Here's the drawing with two shaded views (mm, measured from the low corner). I have some questions. A direction names the side the tool comes from. Coordinates: 2 decimals unless noted, no trailing zeros. Loops run counter-clockwise (first coordinate to the right, second up) from the corner with the lowest first, then second, coordinate; pieces in that order, holes last. Notation, with made-up numbers: (-12.75, 52) -> (-4.75, 52) arc R20 ccw to (-4.75, 90) -> close; hole circle Ø1 at (66.25, 73). An arc over 180 degrees is marked (long way). Answer as a JSON object with one key per item and string values. Group by question number.
Q1. I want a section at A-A on z = 17. Write out the boundary of the cut face in (x, y), then the cut area to 3 significant figures.
Q2. I want a section at C-C on z = 11. Write out the boundary of the cut face in (x, y), then the cut area to 3 significant figures.
Q3. I need wall thicknesses on line 1 (X direction, y = 31, z = 13.5); line 2 (Z direction, x = 5, y = 30); line 3 (Z direction, x = 11.5, y = 23). Which ranges of each line are inside material? Lowest first, please.
Q4. I want a section at D-D on y = 30. Write out the boundary of the cut face in (x, z).
Q5. I'm going to push flat-ended pins straight in: pin 1 (3 mm diameter, centred on x = 6, z = 10.5, fed in from -Y); pin 2 (1.5 mm diameter, centred on x = 15.5, y = 17, fed in from +Z); pin 3 (8 mm diameter, centred on x = 57.5, z = 24, fed in from +Y). Where does each tip first touch, or does it pass through?
Q6. Thinking about a two-plate mould opening in Y: for the marked faces 1, 2, 3 and 4, which applies, released by +Y, released by -Y, zero draft, split by the parting line, or undercut?
Q7. On a 3-axis mill with a long thin cutter (end or side, diameter ignored), from which of +Z, -Z, +X, -X, +Y, -Y can I reach the whole of each face in a straight line? I mean the marked faces 5, 6, 7, 8 and 9. Say none if no direction works.
Q8. I want a section at B-B on x = 30. Write out the boundary of the cut face in (y, z).
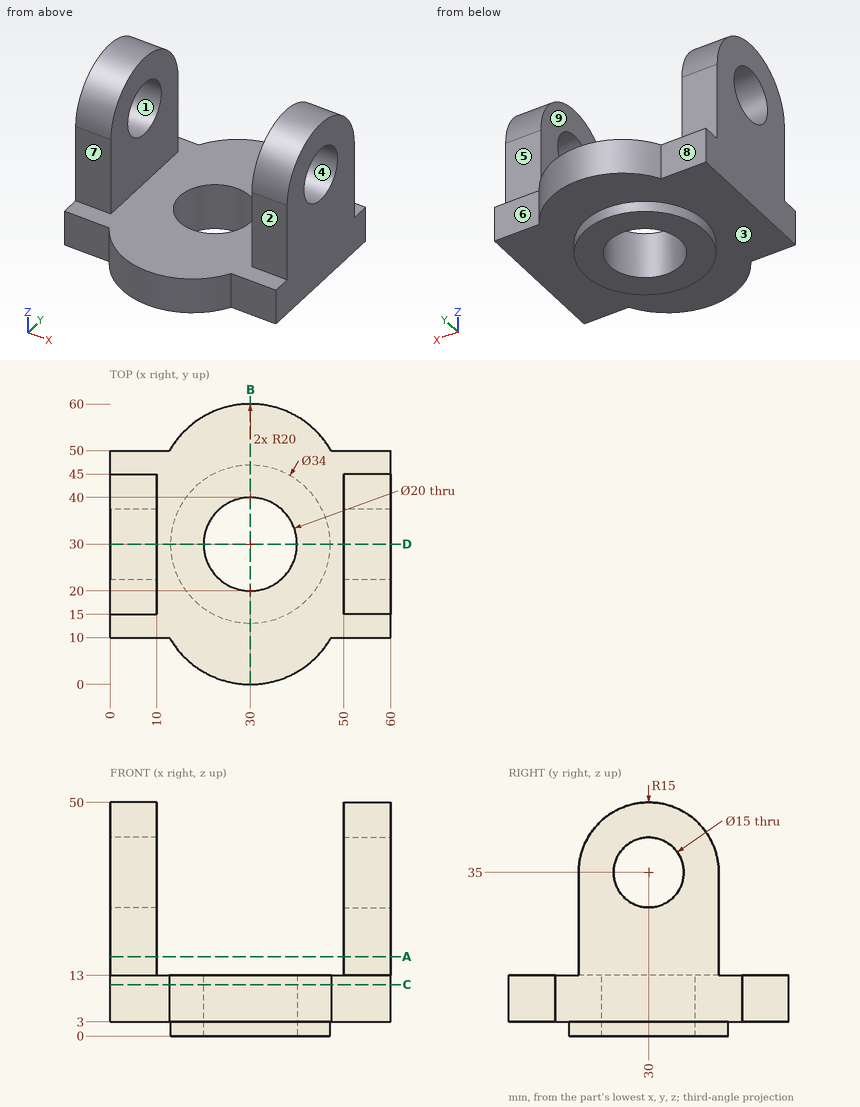
Result set:
{
 "1": {"outline": "(0, 15) -> (10, 15) -> (10, 45) -> (0, 45) -> close; (50, 15) -> (60, 15) -> (60, 45) -> (50, 45) -> close", "area": "600 mm²"},
 "2": {"outline": "(0, 10) -> (12.68, 10) arc R20 ccw to (47.32, 10) -> (60, 10) -> (60, 50) -> (47.32, 50) arc R20 ccw to (12.68, 50) -> (0, 50) -> close; hole circle Ø20 at (30, 30)", "area": "2,580 mm²"},
 "3": {"line 1": "x = 0 to 10, 50 to 60", "line 2": "z = 3 to 27.5, 42.5 to 50", "line 3": "z = 3 to 13"},
 "4": {"outline": "(0, 3) -> (13, 3) -> (13, 0) -> (20, 0) -> (20, 13) -> (10, 13) -> (10, 27.5) -> (0, 27.5) -> close; (0, 42.5) -> (10, 42.5) -> (10, 50) -> (0, 50) -> close; (40, 0) -> (47, 0) -> (47, 3) -> (60, 3) -> (60, 27.5) -> (50, 27.5) -> (50, 13) -> (40, 13) -> close; (50, 42.5) -> (60, 42.5) -> (60, 50) -> (50, 50) -> close"},
 "5": {"pin 1": "stops at y = 10", "pin 2": "stops at z = 13", "pin 3": "stops at y = 45"},
 "6": {"face 1": "undercut", "face 2": "released by -Y", "face 3": "zero draft", "face 4": "undercut"},
 "7": {"face 5": "+Z, +X, -X, +Y", "face 6": "+Z, -Z, +X, +Y", "face 7": "+Z, +X, -X, -Y", "face 8": "+Z, -Z, -X, +Y", "face 9": "+Z, +Y, -Y"},
 "8": {"outline": "(0, 3) -> (13, 3) -> (13, 0) -> (20, 0) -> (20, 13) -> (0, 13) -> close; (40, 0) -> (47, 0) -> (47, 3) -> (60, 3) -> (60, 13) -> (40, 13) -> close"}
}
